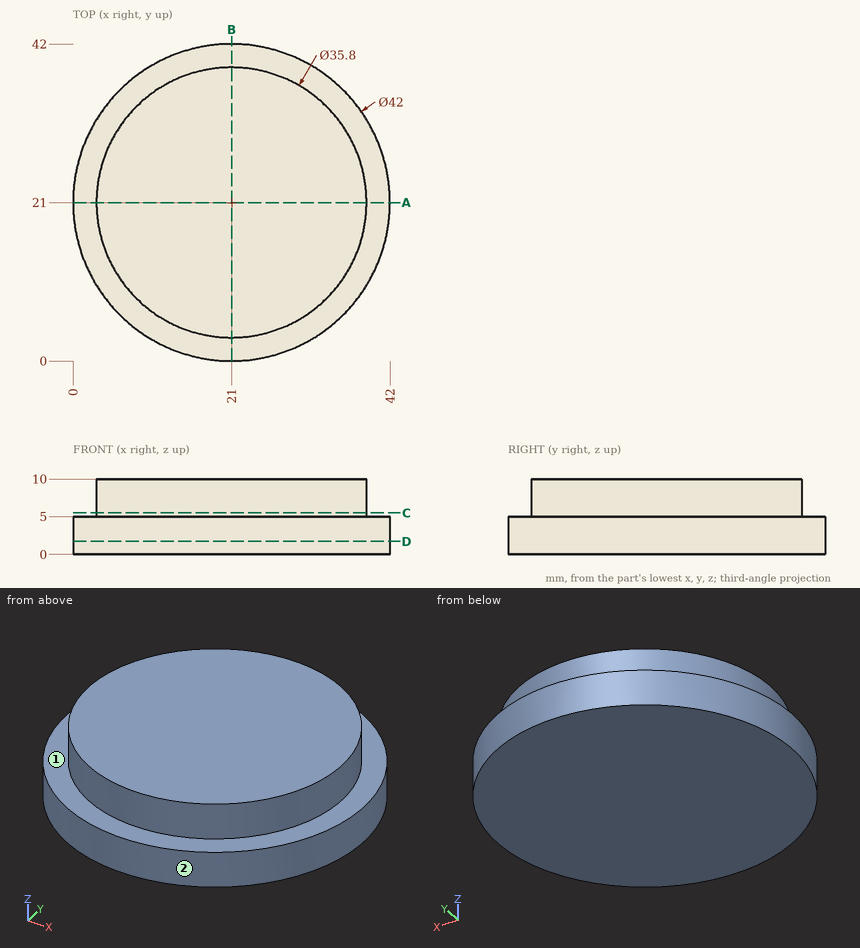
The drawing under review shows one solid part. Ordinate dimensions are in mm from its lowest x, y, z. A direction names the side the tool comes from. Coordinates: 2 decimals unless noted, no trailing zeros. Write each loop counter-clockwise with the first axis right and the second up, starting at its lowest first coordinate (ties: lowest second). Pieces come first, ordered by that corner, then holes. Notation, with made-up numbers: (68, -36.75) - (95, -36.75) arc R25 ccw to (95, 2.25) - close; hole circle Ø4 at (-20.5, 30.5). An arc over 180 degrees is marked (long way). Put each result on its own line as item: value.
1. Machinability: for the marked faces 1 and 2, which of the approach directions +Z, -Z, +X, -X, +Y, -Y give a long, thin tool a straight path to every point of the face, cutting with its end or side? Answer none if there is none.
Values found:
face 1: +Z
face 2: +Z, -Z
2. Add section D-D, the plane z = 1.75. Give the boundary of the cut face in (x, y), then the cut area to 3 significant figures.
Values found:
outline: circle Ø42 at (21, 21)
area: 1,390 mm²
3. Wall thickness on probe 1 along Z at (x, y) = (39, 21); probe 2 along X at (y, z) = (14.5, 8.25); probe 3 along X at (y, z) = (19, 7): over which ranges is each line inside the solid? List them lowest first.
Values found:
probe 1: 0 to 5
probe 2: 4.32 to 37.68
probe 3: 3.21 to 38.79
4. Add section A-A, the plane y = 21. Give the boundary of the cut face in (x, z).
Values found:
outline: (0, 0) - (42, 0) - (42, 5) - (38.9, 5) - (38.9, 10) - (3.1, 10) - (3.1, 5) - (0, 5) - close
5. For pin 1 (3 mm diameter, centred on y = 26.5, z = 2.5, fed in from +X); pin 2 (1.5 mm diameter, centred on x = 6.5, z = 4.5, fed in from +Y); pin 3 (1 mm diameter, centred on x = 30.5, z = 8, fed in from +Y), all flat-tipped, find the tip position at first contact; note any pin that passes through.
Values found:
pin 1: x = 41.62
pin 2: y = 36.87
pin 3: y = 36.47
6. Add section C-C, the plane z = 5.5. Give the boundary of the cut face in (x, y), then the cut area to 3 significant figures.
Values found:
outline: circle Ø35.8 at (21, 21)
area: 1,010 mm²
